from build123d import *

# Parameters (mm, degrees)
BOX017_W               = 115
BOX017_H               = 115
BOX017_DEPTH           = 60
BOX016_W               = 165
BOX016_H               = 165
BOX016_DEPTH           = 45
CUT004_PITCH_ANGLE     = -90
CUT004_PLACEMENT_ANGLE = -90


with BuildPart() as cube013:
    # Box017 → Box017 (new body)
    with BuildSketch(Plane(origin=(25, 25, -7), x_dir=(1, 0, 0), z_dir=(0, 0, 1))):
        with Locations((57.5, 57.5)):
            Rectangle(BOX017_W, BOX017_H)
    extrude(amount=BOX017_DEPTH)


with BuildPart() as bellows:
    # Box016 → Box016 (new body)
    with BuildSketch(Plane.XY):
        with Locations((82.5, 82.5)):
            Rectangle(BOX016_W, BOX016_H)
    extrude(amount=BOX016_DEPTH)

    # Cut004: cut Cube013
    add(cube013.part, mode=Mode.SUBTRACT)


with BuildPart() as bellows_1:
    # Cut004 pitch: moved
    add(bellows.part.rotate(Axis((0, 0, 0), (0, 1, 0)), CUT004_PITCH_ANGLE))


with BuildPart() as bellows_2:
    # Cut004 placement: moved
    add(bellows_1.part.moved(Location((3.5, 14.5, 2))).rotate(Axis((3.5, 14.5, 2), (0, 0, 1)), CUT004_PLACEMENT_ANGLE))


solid = bellows_2.part
Here's how the part is built. I have some questions about the finished solid (model axes, mm). A direction names the side the tool comes from. Coordinates: 2 decimals unless noted, no trailing zeros. Write each loop counter-clockwise with the first axis right and the second up, starting at its lowest first coordinate (ties: lowest second). Pieces come first, ordered by that corner, then holes.
Item 1: If I drill on line 1 (X direction, y = 33, z = 52.5); line 2 (Z direction, x = 87, y = 22), over which ranges is the centre line in solid material (lowest first)?
Item 2: I want a section at A-A on x = 59. Write out the boundary of the cut face in (y, z), and give its area (3 significant figures).
Item 3: On a 3-axis mill with a long thin cutter (end or side, diameter ignored), from which of +Z, -Z, +X, -X, +Y, -Y can I reach the whole of each face in a straight line? I mean faces 4 (the flat face through (85, 37, 2)), 5 (the flat face through (28.5, 37, 84)). Say none if no direction works.
Item 4: I want a section at B-B on z = 117.5. Write out the boundary of the cut face in (x, y).
Item 5: I want a section at C-C on y = 30.5. Write out the boundary of the cut face in (x, z), and give its area (3 significant figures).
Item 6: If we mould it in two halves opening along X, with no side actions, what happens to faces 1 (the flat face through (87, 59.5, 10)), 2 (the flat face through (3.5, 37, 83)), 3 (the flat face through (143.5, 37, 84))? For each: +X half, -X half, draft (parallel to the pull), parting line (faces both ways), or undercut.
Findings below:
1. line 1: x = 3.5 to 28.5, 143.5 to 168.5
1. line 2: z = 2 to 27, 142 to 167
2. outline: (14.5, 2) - (59.5, 2) - (59.5, 27) - (14.5, 27) - close; (14.5, 142) - (59.5, 142) - (59.5, 167) - (14.5, 167) - close
2. area: 2,250 mm2
3. face 4: -Z, +X, -X, +Y, -Y
3. face 5: +Y, -Y
4. outline: (3.5, 14.5) - (28.5, 14.5) - (28.5, 59.5) - (3.5, 59.5) - close; (143.5, 14.5) - (168.5, 14.5) - (168.5, 59.5) - (143.5, 59.5) - close
5. outline: (3.5, 2) - (168.5, 2) - (168.5, 167) - (3.5, 167) - close; hole (28.5, 27) - (143.5, 27) - (143.5, 142) - (28.5, 142) - close
5. area: 14,000 mm2
6. face 1: draft
6. face 2: -X half
6. face 3: undercut
